Design review of the part built by this model. Coordinates are the model's own, in mm. Give positions to 0.01 mm unless a question says otherwise; leave off trailing zeros. Loops run counter-clockwise (first coordinate to the right, second up) from the corner with the lowest first, then second, coordinate; pieces in that order, holes last. Notation, with made-up numbers: (-8, 76) -> (48, 76) arc R7 ccw to (48, 82) -> close; hole circle Ø3 at (14, -33). An arc over 180 degrees is marked (long way). Answer as CSV lines item,"result".
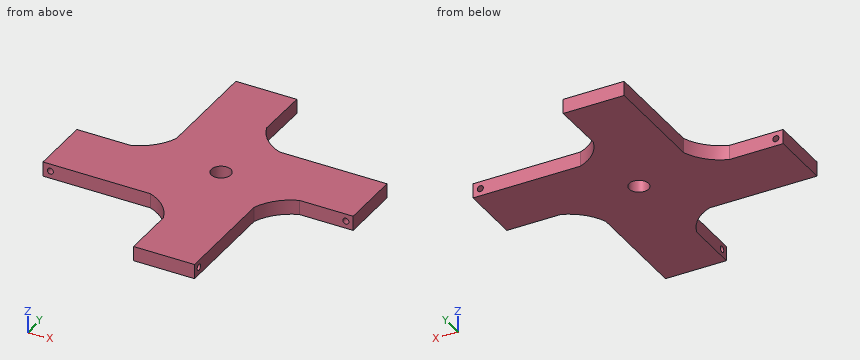
from build123d import *

# Parameters (mm, degrees)
SKETCH_2_R          = 4
EXTRUDE_1_DEPTH     = 6
SKETCH_3_R          = 1.25
CUT_EXTRUDE_1_DEPTH = 5
CUT_EXTRUDE_START   = -5
SKETCH_4_R          = 1.25
CUT_EXTRUDE_2_DEPTH = 5
SKETCH_5_R          = 1.25
CUT_EXTRUDE_3_DEPTH = 5
SKETCH_6_R          = 1.25
CUT_EXTRUDE_4_DEPTH = 5
SKETCH_8_R          = 1.25
CUT_EXTRUDE_5_DEPTH = 5
SKETCH_9_R          = 1.25
CUT_EXTRUDE_6_DEPTH = 5


with BuildPart() as part:
    # 스케치2 → 보스-돌출1 (new body)
    with BuildSketch(Plane.XY):
        with BuildLine():
            Line((-102.525284978, -57.601148056), (-102.525284978, -32.601148056))
            Line((-102.525284978, -32.601148056), (-80.525284978, -32.601148056))
            ThreePointArc((-80.525284978, -32.601148056), (-73.11411316, -27.970582536), (-68.384824454, -20.622015799))
            Line((-68.384824454, -20.622015799), (-68.384824454, 23.377984201))
            Line((-68.384824454, 23.377984201), (-43.384824454, 23.377984201))
            Line((-43.384824454, 23.377984201), (-43.545565494, 1.378571429))
            ThreePointArc((-43.545565494, 1.378571429), (-38.886846868, -5.94242943), (-31.565846009, -10.601148056))
            Line((-31.565846009, -10.601148056), (12.434153991, -10.601148056))
            Line((12.434153991, -10.601148056), (12.434153991, -35.601148056))
            Line((12.434153991, -35.601148056), (-9.565846009, -35.601148056))
            ThreePointArc((-9.565846009, -35.601148056), (-16.886846868, -40.259866682), (-21.545565494, -47.580867541))
            Line((-21.545565494, -47.580867541), (-21.545565494, -91.580867541))
            Line((-21.545565494, -91.580867541), (-46.545565494, -91.580867541))
            Line((-46.545565494, -91.580867541), (-46.545565494, -69.580867541))
            ThreePointArc((-46.545565494, -69.580867541), (-51.20428412, -62.259866682), (-58.525284978, -57.601148056))
            Line((-58.525284978, -57.601148056), (-102.525284978, -57.601148056))
        make_face()
        with Locations((-43.384824454, -32.601148056)):
            Circle(SKETCH_2_R, mode=Mode.SUBTRACT)
    extrude(amount=EXTRUDE_1_DEPTH)

    # 스케치3 → 컷-돌출1 (cut)
    with BuildSketch(Plane(origin=(0, -57.601148056, 0), x_dir=(-1, 0, 0), z_dir=(0, -1, 0))):
        with Locations(Location((99.525284978, -3, 0), (0, 0, 90))):
            Circle(SKETCH_3_R)
    extrude(amount=-CUT_EXTRUDE_1_DEPTH, mode=Mode.SUBTRACT)

    # 스케치4 → 컷-돌출2 (cut)
    with BuildSketch(Plane(origin=(0, -32.601148056, 0), x_dir=(1, 0, 0), z_dir=(0, 1, 0)).offset(CUT_EXTRUDE_START)):
        with Locations(Location((-99.525284978, -3, 0), (0, 0, 90))):
            Circle(SKETCH_4_R)
    extrude(amount=CUT_EXTRUDE_2_DEPTH, mode=Mode.SUBTRACT)

    # 스케치5 → 컷-돌출3 (cut)
    with BuildSketch(Plane(origin=(-21.545565494, 0, 0), x_dir=(0, 0, -1), z_dir=(1, 0, 0))):
        with Locations(Location((-3.087647422, -88.347802665, 0), (0, 0, 90))):
            Circle(SKETCH_5_R)
    extrude(amount=-CUT_EXTRUDE_3_DEPTH, mode=Mode.SUBTRACT)

    # 스케치6 → 컷-돌출4 (cut)
    with BuildSketch(Plane.ZY.offset(46.545565494).offset(CUT_EXTRUDE_START)):
        with Locations(Location((3.087647422, -88.347802665, 0), (0, 0, 90))):
            Circle(SKETCH_6_R)
    extrude(amount=CUT_EXTRUDE_4_DEPTH, mode=Mode.SUBTRACT)

    # 스케치8 → 컷-돌출5 (cut)
    with BuildSketch(Plane(origin=(0, -10.601148056, 0), x_dir=(1, 0, 0), z_dir=(0, 1, 0))):
        with Locations(Location((9.434153991, -3, 0), (0, 0, 180))):
            Circle(SKETCH_8_R)
    extrude(amount=-CUT_EXTRUDE_5_DEPTH, mode=Mode.SUBTRACT)

    # 스케치9 → 컷-돌출6 (cut)
    with BuildSketch(Plane(origin=(0, -35.601148056, 0), x_dir=(-1, 0, 0), z_dir=(0, -1, 0)).offset(CUT_EXTRUDE_START)):
        with Locations((-9.434153991, -3)):
            Circle(SKETCH_9_R)
    extrude(amount=CUT_EXTRUDE_6_DEPTH, mode=Mode.SUBTRACT)


solid = part.part
Q1. We need section B-B, the plane y = -81.5. State the section outline as (x, z) points, and give its area (3 significant figures).
Filled sheet:
outline,"(-46.55, 0) -> (-21.55, 0) -> (-21.55, 6) -> (-46.55, 6) -> close"
area,"150 mm^2"
Q2. We need section A-A, the plane x = 1.5. State the section outline as (y, z) points, and give its area (3 significant figures).
Filled sheet:
outline,"(-35.6, 0) -> (-10.6, 0) -> (-10.6, 6) -> (-35.6, 6) -> close"
area,"150 mm^2"
Q3. Clearance check with flat-ended pins moving along their axes: pin 1 Ø3 at (y, z) = (-88.35, 3.09) entering from -X; pin 2 Ø1.8 at (x, z) = (-15, 4) entering from +Y; pin 3 Ø1 at (y, z) = (11, 1) entering from -X. State where each tip first meets the part, or that it passes through.
Filled sheet:
pin 1,"stops at x = -46.55"
pin 2,"stops at y = -10.6"
pin 3,"stops at x = -68.38"
Q4. We need section C-C, the plane y = -56. State the section outline as (x, z) points.
Filled sheet:
outline,"(-102.53, 0) -> (-21.55, 0) -> (-21.55, 6) -> (-102.53, 6) -> close; hole circle Ø2.5 at (-99.53, 3)"
Q5. To check wall thickness, follow probe 1 along X at (y, z) = (-55, 3); probe 2 along Y at (x, z) = (-61, 3.7); probe 3 along X at (y, z) = (-16, 5). State the ranges of each line that lie inside material, in increasing order. Write a range as from..to.
Filled sheet:
probe 1,"x = -102.53..-100.78, -98.28..-21.55"
probe 2,"y = -57.6..23.38"
probe 3,"x = -68.38..12.43"
